The model under review builds one solid part; all positions refer to its coordinate system, in mm. A direction names the side the tool comes from. Round coordinates to 2 decimals unless told otherwise and drop trailing zeros. Order: outer loops, then holes, each group sorted by start corner. A loop starts at its lowest first (then second) coordinate and runs counter-clockwise, first axis right, second up.
Autodesk Inventor part; units mm, degrees
ref_plane "YZ Plane" through (0, 0, 0) normal (1, 0, 0) x (0, 1, 0)
ref_plane "XZ Plane" through (0, 0, 0) normal (0, 1, 0) x (-1, 0, 0)
ref_plane "XY Plane" through (0, 0, 0) normal (0, 0, 1) x (1, 0, 0)
sketch "スケッチ1" plane through (0, 0, 0) normal (0, 1, 0) x (-1, 0, 0)
  line L0 (-5.0796, -45.5704) -> (-5.0796, 73.9296)
  line L1 (-5.0796, 73.9296) -> (-4.5796, 74.4296)
  line L2 (-4.5796, 74.4296) -> (24.4204, 74.4296)
  line L3 (24.4204, 74.4296) -> (24.9204, 73.9296)
  line L4 (24.9204, 73.9296) -> (24.9204, -45.5704)
  line L5 (24.9204, -45.5704) -> (-5.0796, -45.5704)
  line L6 (1.9204, -47.0704) -> (1.9204, -50.5704)
  line L7 (1.9204, -50.5704) -> (17.9204, -50.5704)
  line L8 (17.9204, -50.5704) -> (17.9204, -47.0704)
  line L9 (17.9204, -47.0704) -> (1.9204, -47.0704)
  line L10 (2.9204, -47.0704) -> (2.9204, -45.5704)
  line L11 (16.9204, -45.5704) -> (16.9204, -47.0704)
  line L12 (31.4204, 56.4296) -> (30.9204, 56.9296)
  line L13 (30.9204, 56.9296) -> (30.9204, 71.9296)
  line L14 (30.9204, 71.9296) -> (31.4204, 72.4296)
  line L15 (31.4204, 72.4296) -> (38.4204, 72.4296)
  line L16 (38.4204, 72.4296) -> (38.9204, 71.9296)
  line L17 (38.9204, 71.9296) -> (38.9204, 56.9296)
  line L18 (38.9204, 56.9296) -> (38.4204, 56.4296)
  line L19 (38.4204, 56.4296) -> (31.4204, 56.4296)
  line L20 (31.4204, 56.4296) -> (31.4204, 72.4296)
  line L21 (30.9204, 70.4296) -> (27.9204, 70.4296)
  line L22 (27.9204, 70.4296) -> (27.9204, 58.4296)
  line L23 (27.9204, 58.4296) -> (30.9204, 58.4296)
  line L24 (38.4204, 56.4296) -> (38.4204, 72.4296)
  line L25 (27.9204, 66.9296) -> (24.9204, 66.9296)
  line L26 (27.4204, 66.9296) -> (27.4204, 61.9296)
  line L27 (27.9204, 61.9296) -> (24.9204, 61.9296)
  line L28 (24.9204, 73.9296) -> (-5.0796, 73.9296)
  line L29 (-5.0796, 97.1797) -> (24.9204, 97.1797)
  line L30 (24.9204, 97.1797) -> (24.9204, 105.1797)
  line L31 (24.9204, 105.1797) -> (-5.0796, 105.1797)
  line L32 (-5.0796, 105.1797) -> (-5.0796, 97.1797)
  line L33 (24.9204, 99.1797) -> (27.9204, 99.1797)
  line L34 (27.2723, 99.1797) -> (27.2723, 103.1797)
  line L35 (27.9204, 103.1797) -> (24.9204, 103.1797)
  line L36 (27.9204, 105.6797) -> (27.9204, 96.6797)
  line L37 (27.9204, 96.6797) -> (28.4204, 96.1797)
  line L38 (28.4204, 96.1797) -> (32.4204, 96.1797)
  line L39 (32.4204, 96.1797) -> (32.9204, 96.6797)
  line L40 (32.9204, 96.6797) -> (32.9204, 105.6797)
  line L41 (32.9204, 105.6797) -> (32.4204, 106.1797)
  line L42 (32.4204, 106.1797) -> (28.4204, 106.1797)
  line L43 (28.4204, 106.1797) -> (27.9204, 105.6797)
  line L44 (28.4204, 106.1797) -> (28.4204, 96.1797)
  line L45 (32.4204, 96.1797) -> (32.4204, 106.1797)
  line L46 (2.4204, -50.5704) -> (2.4204, -47.0704)
  line L47 (-0.0796, -40.5704) -> (-0.0796, 74.4296)
  line L48 (19.9204, 74.4296) -> (19.9204, -40.5704)
  line L49 (19.9204, -40.5704) -> (9.9204, -46.3439)
  line L50 (9.9204, -46.3439) -> (-0.0796, -40.5704)
  line L51 (-0.0796, -40.5704) -> (19.9204, -40.5704)
  line L52 (17.4204, -47.0704) -> (17.4204, -50.5704)
  line L53 (9.9204, -56.5156) -> (9.9204, 78.76)
  line L54 (9.9204, 93.5864) -> (9.9204, 108.5157)
  line L55 (19.9204, 105.1797) -> (19.9204, 97.1797)
  line L56 (22.5096, 101.1797) -> (35.2156, 101.1797)
  line L57 (27.9204, 103.1797) -> (27.2723, 102.4797)
  line L58 (27.2723, 102.4797) -> (24.9204, 102.4797)
  line L59 (24.9204, 99.8797) -> (27.2723, 99.8797)
  line L60 (27.2723, 99.8797) -> (27.9204, 99.1797)
  line L61 (-0.0796, 97.1797) -> (-0.0796, 105.1797)
  line L62 (24.9204, 66.2296) -> (27.4204, 66.2296)
  line L63 (27.4204, 66.2296) -> (27.9204, 66.9296)
  line L64 (27.4204, 62.6296) -> (27.9204, 61.9296)
  line L65 (27.4204, 62.6296) -> (24.9204, 62.6296)
  line L66 (22.6428, 64.4296) -> (42.5049, 64.4296)
  line L67 (32.2954, 71.4296) -> (38.4204, 71.4296)
  line L68 (33.1704, 70.4296) -> (38.4204, 70.4296)
  line L69 (34.0454, 69.4296) -> (38.4204, 69.4296)
  line L70 (34.9204, 68.4296) -> (38.4204, 68.4296)
  line L71 (35.7954, 67.4296) -> (38.4204, 67.4296)
  line L72 (36.6704, 66.4296) -> (38.4204, 66.4296)
  line L73 (37.5454, 65.4296) -> (38.4204, 65.4296)
  line L74 (29.2204, 105.1797) -> (32.4204, 105.1797)
  line L75 (30.0204, 104.1797) -> (32.4204, 104.1797)
  line L76 (30.8204, 103.1797) -> (32.4204, 103.1797)
  line L77 (31.6204, 102.1797) -> (32.4204, 102.1797)
  point P0 (0, 0)
  point P1 (52.3578, -69.094)
  point P2 (52.3578, -59.2279)
  point P3 (9.9204, 74.4296)
  point P4 (9.9204, -45.5704)
  point P5 (11.2601, -45.5704)
  point P6 (9.9204, -46.3439)
  point P7 (9.9204, -50.5704)
  point P8 (24.4204, 74.4296)
revolve "回転1" add sketch "スケッチ1" angle 360 about axis through (-9.9204, 0, -56.5156) along (0, 0, 1) contours L49 L5 L11 L9 L53 | L9 L52 L7 L53 | L48 L2 L3 L28 | L28 L4 L5 L49 L48 | L9 L8 L7 L52
sketch "スケッチ2" plane through (-9.9204, 0, 74.4296) normal (0, 0, 1) x (1, 0, 0)
  line L0 (0, 0) -> (55.7189, 0) construction
  point P0 (9.9204, 0)
ref_plane "作業平面1" through (-9.9204, 0, 74.4296) normal (0, -1, 0) x (1, 0, 0)
sketch "スケッチ3" plane through (-9.9204, 0, 74.4296) normal (0, -1, 0) x (1, 0, 0)
  line L0 (10, 0) -> (-10, 0)
  line L1 (0, 0) -> (0, -10) construction
  circle A0 centre (0, -10) radius 2.5
  point P0 (9.9204, -74.4296)
  dimension "d2" = 10
  dimension "d3" = 5
extrude "押し出し1" cut sketch "スケッチ3" against normal through all
thread "ねじ1"
thread "ねじ2"
properties part number "stand_base" material "UHMW、黒"
(1) For faces 5 (the cylindrical face through (-23.777, -5.745, 13.343)), 6 (the flat face through (-14, 6, -47.07)), 7 (the cylindrical face through (-7.6, 12.3, 63.5)), 8 (the flat face through (-10, 0, -50.57)), list the 3-axis set-ups (+Z, -Z, +X, -X, +Y, -Y) from which the entire face can be reached by the end or side of a thin tool; tool diameter is ignored.
Data:
face 5: +Z, -Z
face 6: none
face 7: +Y
face 8: -Z, +X, -X, +Y, -Y
(2) Insertion check: pin 1 (1 mm diameter, centred on x = -1, y = 5, fed in from -Z); pin 2 (8 mm diameter, centred on x = -12, y = -3, fed in from +Z); pin 3 (6 mm diameter, centred on y = -0.5, z = 40.5, fed in from +X); pin 4 (1 mm diameter, centred on y = 6, z = -29.5, fed in from -X). Each pin has a flat end and moves straight along its axis. Give the tip position at first contact, or say it passes through.
Data:
pin 1: stops at z = -45.57
pin 2: stops at z = -41.93
pin 3: stops at x = 5.08
pin 4: stops at x = -23.88
(3) To check wall thickness, follow probe 1 along X at (y, z) = (0, 45.5); probe 2 along Z at (x, y) = (3, 3); probe 3 along X at (y, z) = (8, 23). State the ranges of each line that lie inside material, in increasing order.
Data:
probe 1: x = -24.92 to -19.92, 0.08 to 5.08
probe 2: z = -45.57 to 74.43
probe 3: x = -22.61 to -15.92, -3.92 to 2.77
(4) Draft analysis for pull direction X (two halves, no side actions). For faces 1 (the cylindrical face through (-19.46, 3, 16.12)), 2 (the cylindrical face through (-8.403, -6.834, -46.331)), 3 (the conical face through (-11.58, -0.52, -45.34)), 4 (the flat face through (-13, -10, 74.43)), state which applies: pulls with the +X half, pulls with the -X half, needs draft (parallel to the pull), parting line crosses it, or undercut.
Data:
face 1: undercut
face 2: parting line crosses it
face 3: undercut
face 4: needs draft
(5) Consider section A-A (z = 39). Write out the cut boundary in (x, y).
Data:
outline: circle Ø30 at (-9.92, 0); hole circle Ø20 at (-9.92, 0)
